Check sheet for the modelled part. Datum: model origin and axes. Units: mm. Face numbers are marked on the shaded views. A direction names the side the tool comes from. Round coordinates to 2 decimals unless told otherwise and drop trailing zeros. Loops run counter-clockwise (first coordinate to the right, second up) from the corner with the lowest first, then second, coordinate; pieces in that order, holes last. Notation, with made-up numbers: M -21.75,31 L 11.25,31 A13 cw 11.25,51 Z; hole C 54,82 d6. An arc over 180 degrees is marked long. Write item = value, one per line. Start each with the question number.
(1) Mould release check, pull along Y, two halves, no side actions. Record for the marked faces 5, 6, 7 and 8: pulls with the +Y half, pulls with the -Y half, needs draft (parallel to the pull), parting line crosses it, or undercut.
(2) Cross-section at D-D on x = 84.5. Record the boundary of the cut face in (y, z), plus the area to 3 significant figures.
(3) Scan lines: L1, parallel to Z at x = -21, y = 28.5; L2, parallel to Y at x = 2.5, z = 61; L3, parallel to Y at x = 45, z = 28. Record each from-to range of solid material in increasing order. Write a range as from..to.
(4) Set-up check for the marked faces 1, 2, 3 and 4: record each of +Z, -Z, +X, -X, +Y, -Y from which the full face is reachable in a straight line by a thin tool's end or side.
(5) Cross-section at C-C on y = 80. Record the boundary of the cut face in (x, z), plus the area to 3 significant figures.
(6) Cross-section at A-A on x = 0. Record the boundary of the cut face in (y, z).
(7) Cross-section at B-B on z = 38. Record the boundary of the cut face in (x, y).
(8) Go/stop test with flat-tipped pins: P1, Ø4.5, axis at x = -57.16, y = 70.63, coming from the -Z side; P2, Ø1, axis at y = 71, z = 59.5, coming from the -X side; P3, Ø12.5, axis at y = 83, z = 26, coming from the -X side. Record where each tip stops, or that it passes through.
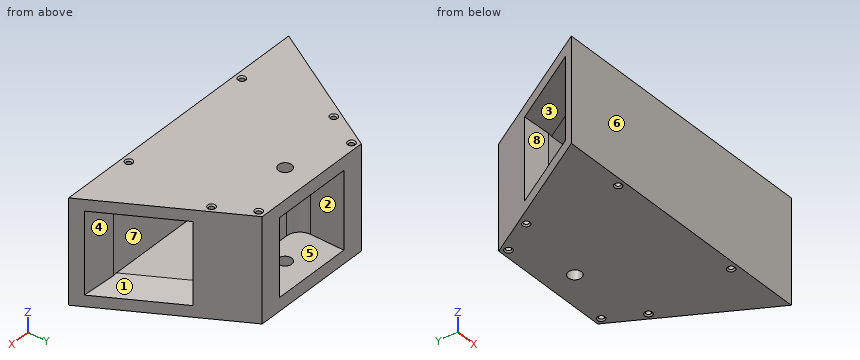
from build123d import *
from OCP.BRepFilletAPI import BRepFilletAPI_MakeChamfer

# Parameters (mm, degrees)
BOSS_EXTRUDE1_DEPTH     = 78
SKETCH3_W               = 54
SKETCH3_H               = 49
CUT_EXTRUDE1_DEPTH      = 164.27356518
CUT_EXTRUDE1_DEPTH_BACK = 164.27356518
CHAMFER1_SIZE           = 20
CHAMFER1_SIZE2          = 4.499551712
CHAMFER1_SIZE2_2        = 3.526539614
CHAMFER1_SIZE2_3        = 3.683833732
CUT_EXTRUDE2_DEPTH      = 164.27356518
SKETCH8_W               = 60
SKETCH8_H               = 46.143990022
SKETCH8_R               = 4.91
BOSS_EXTRUDE4_DEPTH     = 10
BOSS_EXTRUDE5_START     = -78
SKETCH8_3_W             = 60
SKETCH8_3_H             = 46.143990022
SKETCH8_3_R             = 4.91
BOSS_EXTRUDE5_DEPTH     = 10
SKETCH10_R              = 1.85
CUT_EXTRUDE4_DEPTH      = 164.27356518
CHAMFER2_SIZE           = 1


with BuildPart() as part:
    # Sketch2 → Boss-Extrude1 (new body)
    with BuildSketch(Plane.XY):
        Polygon((46.3, 100), (-46.3, 100), (-102.831206773, 0), (102.831206773, 0), align=None)
    extrude(amount=BOSS_EXTRUDE1_DEPTH)

    # Sketch3 → Cut-Extrude1 (cut, two sides)
    with BuildSketch(Plane(origin=(0, 0, 0), x_dir=(0, 0, -1), z_dir=(1, 0, 0))) as cut_extrude1_sk:
        with Locations((-39, 36.5)):
            Rectangle(SKETCH3_W, SKETCH3_H)
    extrude(amount=CUT_EXTRUDE1_DEPTH, mode=Mode.SUBTRACT)
    extrude(cut_extrude1_sk.sketch, amount=-CUT_EXTRUDE1_DEPTH_BACK, mode=Mode.SUBTRACT)

    # Chamfer1: one chamfer whose edges measure the first distance from different faces: ONE call of the kernel's chamfer builder (chamfer() names one face for all edges)
    chamfer1_edges_1 = [part.edges().sort_by_distance(p)[0] for p in [
        (96.04746196, 12, 39),
        (-96.04746196, 12, 39),
    ]]
    chamfer1_side_1 = [part.faces().sort_by_distance(p)[0] for p in [
        (0, 12, 39),
    ]]
    chamfer1_edges_2 = [part.edges().sort_by_distance(p)[0] for p in [
        (82.197316301, 36.5, 12),
        (-82.197316301, 36.5, 12),
    ]]
    chamfer1_side_2 = [part.faces().sort_by_distance(p)[0] for p in [
        (0, 35.123926814, 12),
    ]]
    chamfer1_edges_3 = [part.edges().sort_by_distance(p)[0] for p in [
        (68.347170642, 61, 39),
        (-68.347170642, 61, 39),
    ]]
    chamfer1_side_3 = [part.faces().sort_by_distance(p)[0] for p in [
        (0, 61, 39),
    ]]
    chamfer1_edges_4 = [part.edges().sort_by_distance(p)[0] for p in [
        (82.197316301, 36.5, 66),
        (-82.197316301, 36.5, 66),
    ]]
    chamfer1_side_4 = [part.faces().sort_by_distance(p)[0] for p in [
        (0, 35.123926814, 66),
    ]]
    chamfer1 = BRepFilletAPI_MakeChamfer(part.part.solid().wrapped)
    for e in chamfer1_edges_1:
        chamfer1.Add(CHAMFER1_SIZE, CHAMFER1_SIZE2, e.wrapped, chamfer1_side_1[0].wrapped)  # the first distance lies on this face
    for e in chamfer1_edges_2:
        chamfer1.Add(CHAMFER1_SIZE, CHAMFER1_SIZE2_2, e.wrapped, chamfer1_side_2[0].wrapped)  # the first distance lies on this face
    for e in chamfer1_edges_3:
        chamfer1.Add(CHAMFER1_SIZE, CHAMFER1_SIZE2_3, e.wrapped, chamfer1_side_3[0].wrapped)  # the first distance lies on this face
    for e in chamfer1_edges_4:
        chamfer1.Add(CHAMFER1_SIZE, CHAMFER1_SIZE2_2, e.wrapped, chamfer1_side_4[0].wrapped)  # the first distance lies on this face
    add(Compound.cast(chamfer1.Shape()), mode=Mode.REPLACE)

    # Sketch4 → Cut-Extrude2 (cut, through all)
    with BuildSketch(Plane.XY.offset(78)):
        with BuildLine():
            Line((-20, 65), (20, 65))
            ThreePointArc((20, 65), (27.071067812, 67.928932188), (30, 75))
            Line((30, 75), (30, 100))
            Line((30, 100), (-30, 100))
            Line((-30, 100), (-30, 75))
            ThreePointArc((-30, 75), (-27.071067812, 67.928932188), (-20, 65))
        make_face()
    extrude(amount=-CUT_EXTRUDE2_DEPTH, mode=Mode.SUBTRACT)

    # Sketch8 → Boss-Extrude4 (add)
    with BuildSketch(Plane.XY.offset(78)):
        with Locations((0, 76.928004989)):
            Rectangle(SKETCH8_W, SKETCH8_H)
        with Locations((0, 80)):
            Circle(SKETCH8_R, mode=Mode.SUBTRACT)
    extrude(amount=-BOSS_EXTRUDE4_DEPTH)

    # Sketch8<3> → Boss-Extrude5 (add)
    with BuildSketch(Plane.XY.offset(78).offset(BOSS_EXTRUDE5_START)):
        with Locations((0, 76.928004989)):
            Rectangle(SKETCH8_3_W, SKETCH8_3_H)
        with Locations((0, 80)):
            Circle(SKETCH8_3_R, mode=Mode.SUBTRACT)
    extrude(amount=BOSS_EXTRUDE5_DEPTH)

    # Sketch10 → Cut-Extrude4 (cut, through all)
    with BuildSketch(Plane.XY.offset(78)):
        with Locations((-43.382916604, 95)):
            Circle(SKETCH10_R)
        with Locations((-57.162268727, 70.625229128)):
            Circle(SKETCH10_R)
        with Locations((-52.831206773, 5)):
            Circle(SKETCH10_R)
        with Locations(Location((52.831206773, 5, 0), (0, 0, 180))):
            Circle(SKETCH10_R)
        with Locations(Location((57.162268727, 70.625229128, 0), (0, 0, 180))):
            Circle(SKETCH10_R)
        with Locations(Location((43.382916604, 95, 0), (0, 0, 180))):
            Circle(SKETCH10_R)
    extrude(amount=-CUT_EXTRUDE4_DEPTH, mode=Mode.SUBTRACT)

    # Chamfer2
    chamfer2_edges = [part.edges().sort_by_distance(p)[0] for p in [
        (45.232916604, 95, 0),
        (45.232916604, 95, 78),
        (59.012268727, 70.625229128, 0),
        (59.012268727, 70.625229128, 78),
        (54.681206773, 5, 0),
        (54.681206773, 5, 78),
        (-54.681206773, 5, 0),
        (-54.681206773, 5, 78),
        (-59.012268727, 70.625229128, 0),
        (-59.012268727, 70.625229128, 78),
        (-45.232916604, 95, 0),
        (-45.232916604, 95, 78),
    ]]
    chamfer(chamfer2_edges, length=CHAMFER2_SIZE)


solid = part.part
Result:
q1.face_5 = needs draft
q1.face_6 = pulls with the -Y half
q1.face_7 = undercut
q1.face_8 = undercut
q2.outline = M 0,0 L 32.43,0 L 32.43,8.47 L 10.51,10.38 L 10.51,67.62 L 32.43,69.53 L 32.43,78 L 0,78 Z
q2.area = 1,230 mm^2
q3.L1 = 0..12, 66..78
q3.L2 = 0..12, 61..65
q3.L3 = 0..12, 61..94.1, 95.9..100
q4.face_1 = +X
q4.face_2 = +Y
q4.face_3 = -X
q4.face_4 = +X, +Y
q5.outline = M -57.61,0 L -4.91,0 L -4.91,10 L -30,10 L -30,68 L -4.91,68 L -4.91,78 L -57.61,78 Z; M 4.91,0 L 57.61,0 L 57.61,78 L 4.91,78 L 4.91,68 L 30,68 L 30,10 L 4.91,10 Z
q5.area = 5,310 mm^2
q6.outline = M 0,0 L 75.09,0 L 75.09,10 L 65,10 L 65,68 L 75.09,68 L 75.09,78 L 0,78 Z; M 84.91,0 L 100,0 L 100,10 L 84.91,10 Z; M 84.91,68 L 100,68 L 100,78 L 84.91,78 Z; hole M 12,12 L 61,12 L 61,66 L 12,66 Z
q7.outline = M -102.83,0 L 102.83,0 L 98.26,8.08 L 76.05,12 L -76.05,12 L -98.26,8.08 Z; M -66.53,64.21 L -48.35,61 L 48.35,61 L 66.53,64.21 L 46.3,100 L 30,100 L 30,75 A10 cw 20,65 L -20,65 A10 cw -30,75 L -30,100 L -46.3,100 Z; hole C -57.16,70.63 d3.7; hole C -52.83,5 d3.7; hole C -43.38,95 d3.7; hole C 43.38,95 d3.7; hole C 52.83,5 d3.7; hole C 57.16,70.63 d3.7
q8.P1 = 0.59
q8.P2 = -62.98
q8.P3 = -59.44
